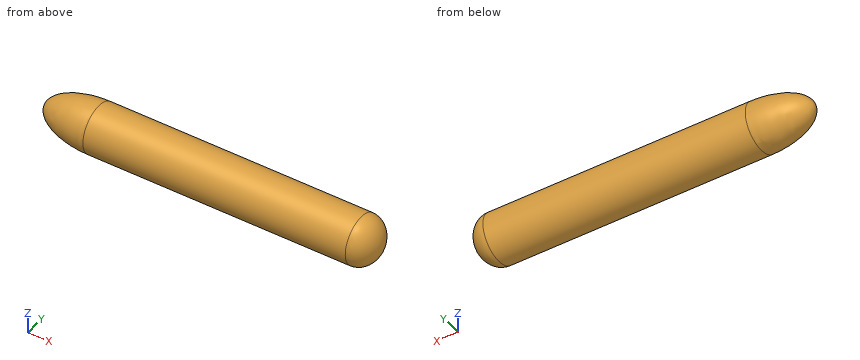
```python
from build123d import *

# Parameters (mm, degrees)
SKETCH1_R           = 115
BOSS_EXTRUDE2_DEPTH = 761.29
BOSS_EXTRUDE3_START = -487.1
SKETCH2_R           = 115
BOSS_EXTRUDE3_DEPTH = 487.1


with BuildPart() as part:
    # Sketch1 → Boss-Extrude2 (new body)
    with BuildSketch(Plane(origin=(0, 0, 0), x_dir=(0, 0, -1), z_dir=(1, 0, 0))):
        Circle(SKETCH1_R)
    extrude(amount=BOSS_EXTRUDE2_DEPTH)

    # Sketch2 → Boss-Extrude3 (add)
    with BuildSketch(Plane(origin=(0, 0, 0), x_dir=(0, 0, -1), z_dir=(1, 0, 0)).offset(BOSS_EXTRUDE3_START)):
        Circle(SKETCH2_R)
    extrude(amount=BOSS_EXTRUDE3_DEPTH)

    # Sketch3 → Revolve1 (revolve)
    with BuildSketch(Plane(origin=(0, 0, 0), x_dir=(1, 0, 0), z_dir=(0, 1, 0))):
        with BuildLine():
            Line((761.29, 0), (858.06, 0))
            add(Edge.make_bspline(
                [(858.06, 0), (858.06, 115), (761.29, 115)],
                knots=[4.71238898, 4.71238898, 4.71238898, 6.283185307, 6.283185307, 6.283185307], degree=2, weights=[1, 0.707106781, 1]))
            Line((761.29, 115), (761.29, 0))
        make_face()
    revolve(axis=Axis((761.29, 0, 0), (1, 0, 0)))

    # Sketch4 → Revolve2 (revolve)
    with BuildSketch(Plane(origin=(0, 0, 0), x_dir=(1, 0, 0), z_dir=(0, 1, 0))):
        with BuildLine():
            Line((-487.1, 0), (-741.94, 0))
            add(Edge.make_bspline(
                [(-741.94, 0), (-741.94, -115), (-487.1, -115)],
                knots=[0, 0, 0, 1.570796327, 1.570796327, 1.570796327], degree=2, weights=[1, 0.707106781, 1]))
            Line((-487.1, -115), (-487.1, 0))
        make_face()
    revolve(axis=Axis((858.06, 0, 0), (-1, 0, 0)))


solid = part.part
```
Can you work these out from the model? Positions are in its coordinate system, mm. Coordinates: 2 decimals unless noted, no trailing zeros. Loops run counter-clockwise (first coordinate to the right, second up) from the corner with the lowest first, then second, coordinate; pieces in that order, holes last. Notation, with made-up numbers: (-23.5, -3) - (1.5, -3) arc R18 cw to (1.5, 1) - close; hole circle Ø5 at (-20.5, 79). An arc over 180 degrees is marked (long way). Use a Markdown table: item, result.
Item 1: If I drill on probe 1 along Z at (x, y) = (-303, 7.5); probe 2 along Y at (x, z) = (557, 2.5); probe 3 along Z at (x, y) = (688.5, 76.5), over which ranges is the centre line in solid material (lowest first)? Write a range as from..to.
Numbers:
| item | result |
|---|---|
| probe 1 | z = -114.76..114.76 |
| probe 2 | y = -114.97..114.97 |
| probe 3 | z = -85.86..85.86 |
Item 2: I want a section at A-A on x = -62.5. Please give me the cut outline in (y, z), and give its area (3 significant figures).
Numbers:
| item | result |
|---|---|
| outline | circle Ø230 at (0, 0) |
| area | 41,500 mm2 |
Item 3: Will these pins go through, and if not, where does the flat tip stop? pin 1 (1 mm diameter, centred on y = -82.5, z = 21, fed in from +X); pin 2 (5 mm diameter, centred on x = 487.5, z = -42, fed in from +Y); pin 3 (2 mm diameter, centred on x = -313, y = 35, fed in from -Z).
Numbers:
| item | result |
|---|---|
| pin 1 | stops at x = 826.81 |
| pin 2 | stops at y = 108 |
| pin 3 | stops at z = -109.86 |
